Design review of the part built by this model. Coordinates are the model's own, in mm. A direction names the side the tool comes from. Coordinates: 2 decimals unless noted, no trailing zeros. Order: outer loops, then holes, each group sorted by start corner. A loop starts at its lowest first (then second) coordinate and runs counter-clockwise, first axis right, second up. Notation, with made-up numbers: M 72,54 L 127,54 A18 cw 127,78 Z; hole C 66,26.5 d8. An arc over 180 degrees is marked long. Answer in a Markdown table with one row per item.
from build123d import *

# Parameters (mm, degrees)
SKETCH1_R               = 3
SKETCH1_R_2             = 2.5
BOSS_EXTRUDE1_DEPTH     = 8
BOSS_EXTRUDE2_START     = 0.25
BOSS_EXTRUDE2_DEPTH     = 7.5
SKETCH4_R               = 4
SKETCH4_R_2             = 3
BOSS_EXTRUDE3_DEPTH     = 2
BOSS_EXTRUDE4_START     = 6
SKETCH4_2_R             = 4
SKETCH4_2_R_2           = 3
BOSS_EXTRUDE4_DEPTH     = 2
CUT_EXTRUDE1_DEPTH      = 10
CUT_EXTRUDE1_DEPTH_BACK = 10
SKETCH6_W               = 1
SKETCH6_H               = 2.845299462


with BuildPart() as part:
    # Sketch1 → Boss-Extrude1 (new body)
    with BuildSketch(Plane(origin=(0, 0, 0), x_dir=(1, 0, 0), z_dir=(0, 1, 0))):
        with Locations(Location((0, 0, 0), (0, 0, 270))):
            Circle(SKETCH1_R)
        with Locations(Location((0, 0, 0), (0, 0, 270))):
            Circle(SKETCH1_R_2, mode=Mode.SUBTRACT)
    extrude(amount=BOSS_EXTRUDE1_DEPTH)

    # Sketch3 → Boss-Extrude2 (add)
    with BuildSketch(Plane(origin=(0, 0, 0), x_dir=(1, 0, 0), z_dir=(0, 1, 0)).offset(BOSS_EXTRUDE2_START)):
        with BuildLine():
            Line((1, 2.291287847), (1, 1.5))
            ThreePointArc((1, 1.5), (1.146446609, 1.146446609), (1.5, 1))
            Line((1.5, 1), (2.291287847, 1))
            ThreePointArc((2.291287847, 1), (1.767766953, 1.767766953), (1, 2.291287847))
        make_face()
        with BuildLine():
            Line((1, -2.291287847), (1, -1.5))
            ThreePointArc((1, -1.5), (1.146446609, -1.146446609), (1.5, -1))
            Line((1.5, -1), (2.291287847, -1))
            ThreePointArc((2.291287847, -1), (1.767766953, -1.767766953), (1, -2.291287847))
        make_face()
        with BuildLine():
            Line((-2.291287847, -1), (-1.5, -1))
            ThreePointArc((-1.5, -1), (-1.146446609, -1.146446609), (-1, -1.5))
            Line((-1, -1.5), (-1, -2.291287847))
            ThreePointArc((-1, -2.291287847), (-1.767766953, -1.767766953), (-2.291287847, -1))
        make_face()
        with BuildLine():
            Line((-1, 2.291287847), (-1, 1.5))
            ThreePointArc((-1, 1.5), (-1.146446609, 1.146446609), (-1.5, 1))
            Line((-1.5, 1), (-2.291287847, 1))
            ThreePointArc((-2.291287847, 1), (-1.767766953, 1.767766953), (-1, 2.291287847))
        make_face()
    extrude(amount=BOSS_EXTRUDE2_DEPTH)

    # Sketch4 → Boss-Extrude3 (add)
    with BuildSketch(Plane(origin=(0, 0, 0), x_dir=(1, 0, 0), z_dir=(0, 1, 0))):
        with Locations(Location((0, 0, 0), (0, 0, 270))):
            Circle(SKETCH4_R)
        with Locations(Location((0, 0, 0), (0, 0, 270))):
            Circle(SKETCH4_R_2, mode=Mode.SUBTRACT)
    extrude(amount=BOSS_EXTRUDE3_DEPTH)

    # Sketch4_2 → Boss-Extrude4 (add)
    with BuildSketch(Plane(origin=(0, 0, 0), x_dir=(1, 0, 0), z_dir=(0, 1, 0)).offset(BOSS_EXTRUDE4_START)):
        with Locations(Location((0, 0, 0), (0, 0, 270))):
            Circle(SKETCH4_2_R)
        with Locations(Location((0, 0, 0), (0, 0, 270))):
            Circle(SKETCH4_2_R_2, mode=Mode.SUBTRACT)
    extrude(amount=BOSS_EXTRUDE4_DEPTH)

    # Sketch5 → Revolve1 (revolve)
    with BuildSketch(Plane(origin=(0, 0, 0), x_dir=(0, 0, -1), z_dir=(1, 0, 0))):
        Polygon((3, 2.577350269), (4, 2), (3, 2), align=None)
        Polygon((3, 6), (4, 6), (3, 5.422649731), align=None)
    revolve(axis=Axis((0, -0.512701632, 0), (0, 1, 0)))

    # Sketch6 → Cut-Extrude1 (cut, two sides: drawn at the far end of the back side and taken through both)
    with BuildSketch(Plane(origin=(0, 0, 0), x_dir=(0, 0, -1), z_dir=(1, 0, 0)).offset(-CUT_EXTRUDE1_DEPTH_BACK)):
        with Locations((0, 4)):
            Rectangle(SKETCH6_W, SKETCH6_H)
    extrude(amount=CUT_EXTRUDE1_DEPTH + CUT_EXTRUDE1_DEPTH_BACK, mode=Mode.SUBTRACT)


solid = part.part
(1) For faces 4 (the cylindrical face through (0, 4, -3)), 5 (the flat face through (2, 0, 2)), 6 (the flat face through (1.5, 0.25, 1.5)), 7 (the flat face through (-1.5, 7.75, -1.5)), list the 3-axis set-ups (+Z, -Z, +X, -X, +Y, -Y) from which the entire face can be reached by the end or side of a thin tool; tool diameter is ignored.
Return value:
| item | result |
|---|---|
| face 4 | -Z |
| face 5 | +Z, -Z, +X, -X, -Y |
| face 6 | -Y |
| face 7 | +Y |
(2) Insertion check: pin 1 Ø1 at (x, z) = (-1.5, -1.5) entering from -Y; pin 2 Ø0.6 at (x, y) = (2.5, 4.5) entering from -Z; pin 3 Ø1 at (x, y) = (-1.5, 1.5) entering from -Z; pin 4 Ø0.9 at (x, y) = (2, 4.5) entering from +Z. Each pin has a flat end and moves straight along its axis. Give the tip position at first contact, or say it passes through.
Return value:
| item | result |
|---|---|
| pin 1 | stops at y = 0 |
| pin 2 | stops at z = -2.04 |
| pin 3 | stops at z = -3.87 |
| pin 4 | stops at z = 2.57 |
(3) Add section C-C, the plane y = 3.25. Give the boundary of the cut face in (x, z).
Return value:
| item | result |
|---|---|
| outline | M -2.96,-0.5 A3 ccw 2.96,-0.5 L 2.45,-0.5 A2.5 cw 2.29,-1 L 1.5,-1 A0.5 ccw 1,-1.5 L 1,-2.29 A2.5 cw -1,-2.29 L -1,-1.5 A0.5 ccw -1.5,-1 L -2.29,-1 A2.5 cw -2.45,-0.5 Z; M -2.96,0.5 L -2.45,0.5 A2.5 cw -2.29,1 L -1.5,1 A0.5 ccw -1,1.5 L -1,2.29 A2.5 cw 1,2.29 L 1,1.5 A0.5 ccw 1.5,1 L 2.29,1 A2.5 cw 2.45,0.5 L 2.96,0.5 A3 ccw Z |
(4) Draft analysis for pull direction Z (two halves, no side actions). For faces 1 (the cylindrical face through (0, 4, 3)), 2 (the cylindrical face through (-3.905, 0.986, -0.867)), 3 (the flat face through (1.5, 7.75, -1.5)), state which applies: pulls with the +Z half, pulls with the -Z half, needs draft (parallel to the pull), parting line crosses it, or undercut.
Return value:
| item | result |
|---|---|
| face 1 | pulls with the +Z half |
| face 2 | parting line crosses it |
| face 3 | undercut |
(5) Add section D-D, the plane z = 0. Give the boundary of the cut face in (x, y).
Return value:
| item | result |
|---|---|
| outline | M -4,0 L -2.5,0 L -2.5,2.58 L -3,2.58 L -4,2 Z; M -4,6 L -3,5.42 L -2.5,5.42 L -2.5,8 L -4,8 Z; M 2.5,0 L 4,0 L 4,2 L 3,2.58 L 2.5,2.58 Z; M 2.5,5.42 L 3,5.42 L 4,6 L 4,8 L 2.5,8 Z |
(6) For line 1 along Y through (x, z) = (2.5, 3); line 2 along X through (y, z) = (7.5, 1.5); line 3 along X through (y, z) = (5.5, 0), list the stretches that pass through material, from the lowest coordinate up. Write a range as from..to.
Return value:
| item | result |
|---|---|
| line 1 | y = 0..2.05, 5.95..8 |
| line 2 | x = -3.71..-1, 1..3.71 |
| line 3 | x = -3.13..-2.5, 2.5..3.13 |
(7) Add section A-A, the plane x = 0. Give the boundary of the cut face in (y, z).
Return value:
| item | result |
|---|---|
| outline | M 0,-4 L 2,-4 L 2.58,-3 L 5.42,-3 L 6,-4 L 8,-4 L 8,-2.5 L 0,-2.5 Z; M 0,2.5 L 8,2.5 L 8,4 L 6,4 L 5.42,3 L 2.58,3 L 2,4 L 0,4 Z |
(8) Add section B-B, the plane y = 0.75. Give the boundary of the cut face in (x, z).
Return value:
| item | result |
|---|---|
| outline | C 0,0 d8; hole M -2.29,-1 L -1.5,-1 A0.5 cw -1,-1.5 L -1,-2.29 A2.5 ccw 1,-2.29 L 1,-1.5 A0.5 cw 1.5,-1 L 2.29,-1 A2.5 ccw 2.29,1 L 1.5,1 A0.5 cw 1,1.5 L 1,2.29 A2.5 ccw -1,2.29 L -1,1.5 A0.5 cw -1.5,1 L -2.29,1 A2.5 ccw Z |
